Design review of the part built by this model. Coordinates are the model's own, in mm. A direction names the side the tool comes from. Round coordinates to 2 decimals unless told otherwise and drop trailing zeros. Loops run counter-clockwise (first coordinate to the right, second up) from the corner with the lowest first, then second, coordinate; pieces in that order, holes last. Notation, with made-up numbers: (-30, 50.5) - (22, 50.5) arc R32 cw to (22, 78.5) - close; hole circle Ø2 at (62.5, -17.5). An arc over 180 degrees is marked (long way). Return JSON: item names as keys, results as strings. Group by question number.
from build123d import *

# Parameters (mm, degrees)
SKETCH_R     = 1.5
PAD_DEPTH    = 3
SKETCH001_W  = 16.5
SKETCH001_H  = 28
SKETCH001_R  = 1.5
PAD001_DEPTH = 3
SKETCH002_R  = 2.5
POCKET_DEPTH = 28.001
FILLET_R     = 1
FILLET001_R  = 1
FILLET002_R  = 1
FILLET003_R  = 1


with BuildPart() as part:
    # Sketch → Pad (new body)
    with BuildSketch(Plane.XY):
        with BuildLine():
            ThreePointArc((-6, 0), (0, -6), (6, 0))
            Line((6, 0), (6, 12.5))
            Line((6, 12.5), (22.5, 12.5))
            Line((22.5, 12.5), (22.5, -15.5))
            Line((-12.5, -15.5), (22.5, -15.5))
            Line((-12.5, 12.5), (-12.5, -15.5))
            Line((-6, 12.5), (-12.5, 12.5))
            Line((-6, 12.5), (-6, 0))
        make_face()
        with Locations((-8.5, -8.5)):
            Circle(SKETCH_R, mode=Mode.SUBTRACT)
        with Locations((8.5, -8.5)):
            Circle(SKETCH_R, mode=Mode.SUBTRACT)
        with Locations((-8.5, 8.5)):
            Circle(SKETCH_R, mode=Mode.SUBTRACT)
        with Locations((8.5, 8.5)):
            Circle(SKETCH_R, mode=Mode.SUBTRACT)
        with Locations((18.5, 8.5)):
            Circle(SKETCH_R, mode=Mode.SUBTRACT)
        with Locations((18.5, -8.5)):
            Circle(SKETCH_R, mode=Mode.SUBTRACT)
    extrude(amount=PAD_DEPTH)

    # Sketch001 → Pad001 (join)
    with BuildSketch(Plane.XY.offset(3)):
        with Locations((14.25, -1.5)):
            Rectangle(SKETCH001_W, SKETCH001_H)
        with Locations((8.5, 8.5)):
            Circle(SKETCH001_R, mode=Mode.SUBTRACT)
        with Locations((18.5, 8.5)):
            Circle(SKETCH001_R, mode=Mode.SUBTRACT)
        with Locations((18.5, -8.5)):
            Circle(SKETCH001_R, mode=Mode.SUBTRACT)
        with Locations((8.5, -8.5)):
            Circle(SKETCH001_R, mode=Mode.SUBTRACT)
    extrude(amount=PAD001_DEPTH)

    # Sketch002 (on Face20 of Pad001) → Pocket (cut, through all)
    with BuildSketch(Plane.XZ.offset(15.5)):
        with Locations((13.5, 6.1)):
            Circle(SKETCH002_R)
    extrude(amount=-POCKET_DEPTH, mode=Mode.SUBTRACT)

    # Fillet
    fillet_edges = [part.edges().sort_by_distance(p)[0] for p in [
        (-12.5, -15.5, 1.5),
        (22.5, -15.5, 1.5),
        (22.5, -15.5, 4.5),
    ]]
    fillet(fillet_edges, radius=FILLET_R)

    # Fillet001
    fillet001_edges = [part.edges().sort_by_distance(p)[0] for p in [
        (-12.5, 12.5, 1.5),
    ]]
    fillet(fillet001_edges, radius=FILLET001_R)

    # Fillet002
    fillet002_edges = [part.edges().sort_by_distance(p)[0] for p in [
        (6, 12.5, 4.5),
        (6, 12.5, 1.5),
    ]]
    fillet(fillet002_edges, radius=FILLET002_R)

    # Fillet003
    fillet003_edges = [part.edges().sort_by_distance(p)[0] for p in [
        (22.5, 12.5, 4.5),
        (22.5, 12.5, 1.5),
    ]]
    fillet(fillet003_edges, radius=FILLET003_R)


solid = part.part
Q1. For line 1 (Y direction, x = 8.5, z = 3.65); line 2 (X direction, y = 3.75, z = 1); line 3 (Z direction, x = -4.5, y = -5.25), list the stretches that pass through material, from the lowest coordinate up.
Q2. Tool access review of faces 1 (the flat face through (-5, -4, 3)), 2 (the cylindrical face through (-9.7, 7.6, 1.5)): name each direction out of +Z, -Z, +X, -X, +Y, -Y from which nothing blocks a thin tool from reaching the whole face with its end or side.
Q3. Add section A-A, the plane x = 8.5. State the section outline as (y, z) points, plus the area to 3 significant figures.
Q4. Add section B-B, the plane y = 2.25. State the section outline as (x, z) points, plus the area to 3 significant figures.
Q5. Add section D-D, the plane y = -8.5. State the section outline as (x, z) points, plus the area to 3 significant figures.
Q6. Add section C-C, the plane y = 8.5. State the section outline as (x, z) points.
Q7. Draft analysis for pull direction Y (two halves, no side actions). For faces 3 (the flat face through (-6, 6, 1)), 4 (the flat face through (8, -15.5, 2)), 5 (the cylindrical face through (7.3, -9.4, 3)), state which applies: pulls with the +Y half, pulls with the -Y half, needs draft (parallel to the pull), parting line crosses it, or undercut.
Q8. Insertion check: pin 1 Ø1 at (y, z) = (-0.5, 5.5) entering from -X; pin 2 Ø5.5 at (x, y) = (-8, -4.5) entering from +Z. Each pin has a flat end and moves straight along its axis. Give the tip position at first contact, or say it passes through.
Evaluation:
{
 "1": {"line 1": "-15.5 to -10, -7 to 7, 10 to 12.5", "line 2": "-12.5 to -6, 6 to 22.5", "line 3": "0 to 3"},
 "2": {"face 1": "+Z, -X, +Y, -Y", "face 2": "+Z, -Z"},
 "3": {"outline": "(-15.5, 0) - (-10, 0) - (-10, 6) - (-15.5, 6) - close; (-7, 0) - (7, 0) - (7, 6) - (-7, 6) - close; (10, 0) - (12.5, 0) - (12.5, 6) - (10, 6) - close", "area": "132 mm²"},
 "4": {"outline": "(-12.5, 0) - (-6, 0) - (-6, 3) - (-12.5, 3) - close; (6, 0) - (22.5, 0) - (22.5, 6) - (16, 6) arc R2.5 cw to (11, 6) - (6, 6) - close", "area": "109 mm²"},
 "5": {"outline": "(-12.5, 0) - (-10, 0) - (-10, 3) - (-12.5, 3) - close; (-7, 0) - (7, 0) - (7, 6) - (6, 6) - (6, 3) - (-7, 3) - close; (10, 0) - (17, 0) - (17, 6) - (16, 6) arc R2.5 cw to (11, 6) - (10, 6) - close; (20, 0) - (22.5, 0) - (22.5, 6) - (20, 6) - close", "area": "100 mm²"},
 "6": {"outline": "(-12.5, 0) - (-10, 0) - (-10, 3) - (-12.5, 3) - close; (-7, 0) - (-6, 0) - (-6, 3) - (-7, 3) - close; (6, 0) - (7, 0) - (7, 6) - (6, 6) - close; (10, 0) - (17, 0) - (17, 6) - (16, 6) arc R2.5 cw to (11, 6) - (10, 6) - close; (20, 0) - (22.5, 0) - (22.5, 6) - (20, 6) - close"},
 "7": {"face 3": "needs draft", "face 4": "pulls with the -Y half", "face 5": "undercut"},
 "8": {"pin 1": "x = 6", "pin 2": "z = 3"}
}
